Input: part model. Units: mm. Frame: model coordinates. A direction names the side the tool comes from. Round coordinates to 2 decimals unless told otherwise and drop trailing zeros. Loops run counter-clockwise (first coordinate to the right, second up) from the corner with the lowest first, then second, coordinate; pieces in that order, holes last.
1) Section A-A, the plane z = 0. Return loops of the section in (x, y).
2) Access query for faces 1 (the face through (-5, 17, -9)), 2 (the face through (2.05, 20, -23)), 3 (the face through (-31.46, 5.91, 20.53)), 4 (the face through (2.05, 6, -37)). Directions: +Z, -Z, +X, -X, +Y, -Y. A direction counts if a zero-diameter tool reaches every point of the face in a straight line with its end or side. Return the directions, or none.
3) First-contact query: pin 1 (2 mm diameter, centred on x = 25.5, y = 11, fed in from -Z); pin 2 (2 mm diameter, centred on y = 22, z = -1, fed in from +X); pin 3 (2.5 mm diameter, centred on y = 6, z = -37.5, fed in from -X). Flat tips, straight axial feed; report the tip coordinate or a pass-through.
4) Ray query, line 1 along X through (y, z) = (3, 0); line 2 along X through (y, z) = (24, 11); line 3 along X through (y, z) = (21.5, -7.5). Return the intervals inside material, ascending.
5) Draft query along Z for faces 5 (the face through (21.66, 16.5, 4.81)), 6 (the face through (18, 0, 27)). Return one class per face: pulls with the +Z half, pulls with the -Z half, needs draft (parallel to the pull), parting line crosses it, or undercut.
6) Section B-B, the plane y = 3. State how many separate pieces and enclosed holes the cut face has, and give its area (3 significant figures).
7) Section C-C, the plane y = 19. Return loops of the section in (x, z).
from build123d import *

# Parameters (mm, degrees)
SKETCH_2_R               = 10
SKETCH_2_R_2             = 1.6
SKETCH_2_W               = 4.1
SKETCH_2_H               = 6.1
CUT_EXTRUDE_1_DEPTH      = 42
SKETCH_3_R               = 1.475
CUT_EXTRUDE_2_DEPTH      = 15
PATTERN_CIRCULAR_1_COUNT = 3


with BuildPart() as part:
    # 草图1 → 旋转1 (revolve)
    with BuildSketch(Plane(origin=(0, 0, 0), x_dir=(0, 0, -1), z_dir=(1, 0, 0)), mode=Mode.PRIVATE) as revolve_1_sk:
        Polygon((0, 25), (-25, 25), (-40, 10), (-40, 0), (-32, 0), (-32, 6.686291501), (-21.686291501, 17), (0, 17), align=None)
    revolve(revolve_1_sk.sketch.rotate(Axis((0, 0, 0), (0, 1, 0)), 180), axis=Axis((0, 0, 0), (0, 1, 0)))

    # 草图2 → 切除-拉伸1 (cut)
    with BuildSketch(Plane(origin=(0, 25, 0), x_dir=(1, 0, 0), z_dir=(0, 1, 0))):
        with Locations(Location((0, 0, 0), (0, 0, 270))):
            Circle(SKETCH_2_R)
        with Locations(Location((12.990381057, 7.5, 0), (0, 0, 270))):
            Circle(SKETCH_2_R_2)
        with Locations(Location((0, -15, 0), (0, 0, 270))):
            Circle(SKETCH_2_R_2)
        with Locations(Location((-12.990381057, 7.5, 0), (0, 0, 270))):
            Circle(SKETCH_2_R_2)
        Polygon((36.618644096, -18.774647922), (31.335889132, -15.724647922), (29.285889132, -19.275352078), (34.568644096, -22.325352078), align=None)
        with Locations((0, 23.05)):
            Rectangle(SKETCH_2_W, SKETCH_2_H)
        with Locations((0, 38.05)):
            Rectangle(SKETCH_2_W, SKETCH_2_H)
        Polygon((18.345508076, -8.224647922), (23.628263039, -11.274647922), (21.578263039, -14.825352078), (16.295508076, -11.775352078), align=None)
        Polygon((-34.568644096, -22.325352078), (-29.285889132, -19.275352078), (-31.335889132, -15.724647922), (-36.618644096, -18.774647922), align=None)
        Polygon((-16.295508076, -11.775352078), (-21.578263039, -14.825352078), (-23.628263039, -11.274647922), (-18.345508076, -8.224647922), align=None)
    extrude(amount=-CUT_EXTRUDE_1_DEPTH, mode=Mode.SUBTRACT)

    # 草图3 → 切除-拉伸2 (cut)
    with BuildSketch(Plane.XY.offset(40)):
        with Locations((0, 3)):
            Circle(SKETCH_3_R)
    cut_extrude_2 = extrude(amount=-CUT_EXTRUDE_2_DEPTH, mode=Mode.SUBTRACT)

    # 阵列(圆周)1: 切除-拉伸2 ×3 about axis
    pattern_circular_1_axis = Axis((0, 10, 0), (0, -1, 0))
    for i in range(1, PATTERN_CIRCULAR_1_COUNT):
        add(cut_extrude_2.rotate(pattern_circular_1_axis, i * 360 / PATTERN_CIRCULAR_1_COUNT), mode=Mode.SUBTRACT)


solid = part.part
Final values:
1. outline: (-40, 0) - (-32, 0) - (-32, 6.69) - (-21.69, 17) - (-10, 17) - (-10, 25) - (-25, 25) - (-40, 10) - close; (10, 17) - (21.69, 17) - (32, 6.69) - (32, 0) - (40, 0) - (40, 10) - (25, 25) - (10, 25) - close
2. face 1: -Y
2. face 2: +Y, -Y
2. face 3: -X, +Y, -Y
2. face 4: -Z, +Y, -Y
3. pin 1: stops at z = -31.05
3. pin 2: stops at x = 28.98
3. pin 3: stops at x = -16.91
4. line 1: x = -40 to -32, 32 to 40
4. line 2: x = -23.56 to -23.15, -16.74 to 16.74, 23.15 to 23.56
4. line 3: x = -27.5 to -14.59, -11.39 to -6.61, 6.61 to 11.39, 14.59 to 27.5
5. face 5: undercut
5. face 6: needs draft
6. separate pieces: 3
6. enclosed holes: 0
6. area: 1,680 mm2
7. outline: circle Ø62 at (0, 0); hole (-23.63, 11.27) - (-18.35, 8.22) - (-16.3, 11.78) - (-21.58, 14.83) - close; hole circle Ø3.2 at (-12.99, -7.5); hole circle Ø20 at (0, 0); hole (-2.05, -26.1) - (2.05, -26.1) - (2.05, -20) - (-2.05, -20) - close; hole circle Ø3.2 at (0, 15); hole circle Ø3.2 at (12.99, -7.5); hole (16.3, 11.78) - (18.35, 8.22) - (23.63, 11.27) - (21.58, 14.83) - close
